Geometry check sheet. Reference: the model listing, model coordinates, mm. A direction names the side the tool comes from. Round coordinates to 2 decimals unless told otherwise and drop trailing zeros. Write each loop counter-clockwise with the first axis right and the second up, starting at its lowest first coordinate (ties: lowest second). Pieces come first, ordered by that corner, then holes. Notation, with made-up numbers: (59.5, -31) -> (69.5, -31) arc R20 cw to (69.5, -1) -> close; hole circle Ø11 at (30, 11). An arc over 180 degrees is marked (long way). Use a Markdown table: item, result.
```python
from build123d import *

# Parameters (mm, degrees)
EXTRUDE_1_DEPTH = 4
SKETCH_2_R      = 1.5
EXTRUDE_2_DEPTH = 5
EXTRUDE_3_DEPTH = 15


with BuildPart() as part:
    # 草图1 → 凸台-拉伸1 (new body)
    with BuildSketch(Plane(origin=(0, 0, 0), x_dir=(1, 0, 0), z_dir=(0, 1, 0))):
        with BuildLine():
            Line((-0.173205081, 4.7), (-4.156921938, -2.2))
            ThreePointArc((-4.156921938, -2.2), (-4.156921938, -2.4), (-3.983716857, -2.5))
            Line((-3.983716857, -2.5), (3.983716857, -2.5))
            ThreePointArc((3.983716857, -2.5), (4.156921938, -2.4), (4.156921938, -2.2))
            Line((4.156921938, -2.2), (0.173205081, 4.7))
            ThreePointArc((0.173205081, 4.7), (0, 4.8), (-0.173205081, 4.7))
        make_face()
    extrude(amount=EXTRUDE_1_DEPTH)

    # 草图2 → 凸台-拉伸2 (add)
    with BuildSketch(Plane.XZ):
        with Locations(Location((0, 0, 0), (0, 0, 90))):
            Circle(SKETCH_2_R)
    extrude(amount=EXTRUDE_2_DEPTH)

    # 草图3 → 凸台-拉伸3 (add)
    with BuildSketch(Plane.XZ.offset(5)):
        Polygon((-1.982050808, -0.566987298), (0.974744871, 1.140119483), (1.474744871, 0.274094079), (-1.482050808, -1.433012702), align=None)
    extrude(amount=EXTRUDE_3_DEPTH)


solid = part.part
```
(1) Release check for a two-part mould opening along Y. For faces 1 (the face through (-1.5, -5, -0.8)), 2 (the face through (2.193, 1.972, -1.202)), 3 (the face through (0, 4, 0)), 4 (the face through (0.5, -5, -0.8)) record: +Y half, -Y half, draft (parallel to the pull), parting line (faces both ways), or undercut.
A:
| item | result |
|---|---|
| face 1 | undercut |
| face 2 | draft |
| face 3 | +Y half |
| face 4 | -Y half |
(2) Thickness scan on line 1 (Y direction, x = 0.5, z = -4); line 2 (Y direction, x = 0.75, z = -1); line 3 (Z direction, x = 1, y = 3). Record the ranges inside material, lowest first.
A:
| item | result |
|---|---|
| line 1 | y = 0 to 4 |
| line 2 | y = -5 to 4 |
| line 3 | z = -3.27 to 2.5 |
(3) Section check D-D on y = -5.25. Record the cut outline in (x, z), plus the area to 3 significant figures.
A:
| item | result |
|---|---|
| outline | (-1.98, -0.57) -> (-1.48, -1.43) -> (1.47, 0.27) -> (0.97, 1.14) -> close |
| area | 3.41 mm2 |
(4) Section check B-B on y = 1.5. Record the cut outline in (x, z), plus the area to 3 significant figures.
A:
| item | result |
|---|---|
| outline | (-4.16, 2.2) -> (-0.17, -4.7) arc R0.2 ccw to (0.17, -4.7) -> (4.16, 2.2) arc R0.2 ccw to (3.98, 2.5) -> (-3.98, 2.5) arc R0.2 ccw to start |
| area | 32.4 mm2 |
(5) Access from +Z, -Z, +X, -X, +Y, -Y to the whole of each face (thin tool, end or side, straight path). Record for faces 5 (the face through (-1, -12, 0)), 6 (the face through (1.221, -12.395, 0.713)), 7 (the face through (0.017, -12.395, -0.568)), 8 (the face through (-1.729, -12.395, -1.006)).
A:
| item | result |
|---|---|
| face 5 | +Z, -X, -Y |
| face 6 | +Z, +X, -Y |
| face 7 | -Z, +X, -Y |
| face 8 | -Z, -X, -Y |
(6) Gauge pin test, flat ends, axial feed: pin 1 Ø1.5 at (y, z) = (-16, -1) entering from +X; pin 2 Ø1.5 at (x, y) = (3.5, -2) entering from +Z; pin 3 Ø2 at (y, z) = (-17, -1) entering from +X. Record the tip position at first contact, or that the pin passes through.
A:
| item | result |
|---|---|
| pin 1 | stops at x = 0.57 |
| pin 2 | passes through |
| pin 3 | stops at x = 1 |
(7) Section check A-A on z = 0. Record the cut outline in (x, y), plus the area to 3 significant figures.
A:
| item | result |
|---|---|
| outline | (-2.89, 0) -> (-1.5, 0) -> (-1.5, -5) -> (-1, -5) -> (-1, -20) -> (1, -20) -> (1, -5) -> (1.5, -5) -> (1.5, 0) -> (2.89, 0) -> (2.89, 4) -> (-2.89, 4) -> close |
| area | 68.1 mm2 |
(8) Section check C-C on x = -3. Record the cut outline in (y, z), plus the area to 3 significant figures.
A:
| item | result |
|---|---|
| outline | (0, 0.2) -> (4, 0.2) -> (4, 2.5) -> (0, 2.5) -> close |
| area | 9.22 mm2 |
